Verification items for the finished model (mm, model axes). Face numbers are marked on the shaded views. A direction names the side the tool comes from. Round coordinates to 2 decimals unless told otherwise and drop trailing zeros. Loops run counter-clockwise (first coordinate to the right, second up) from the corner with the lowest first, then second, coordinate; pieces in that order, holes last. Notation, with made-up numbers: (27, 72.5) -> (80, 72.5) arc R17 ccw to (80, 88.5) -> close; hole circle Ø10 at (86.25, 54.5). An arc over 180 degrees is marked (long way). Use CSV: the item, a comma, the result in double quotes. Start each with the question number.
```python
from build123d import *

# Parameters (mm, degrees)
EXTRUDE_1_DEPTH     = 10
SKETCH_2_W          = 24
SKETCH_2_H          = 25
EXTRUDE_2_DEPTH     = 12
EXTRUDE_3_DEPTH     = 11
CUT_EXTRUDE_1_DEPTH = 15
SKETCH_5_W          = 15
SKETCH_5_H          = 17
CUT_EXTRUDE_2_DEPTH = 1
FILLET_2_R          = 12
FILLET_3_R          = 5
SKETCH_6_R          = 2.1
CUT_EXTRUDE_3_DEPTH = 30
CUT_EXTRUDE_START   = -15
SKETCH_7_R          = 3.5
CUT_EXTRUDE_4_DEPTH = 10


with BuildPart() as part:
    # 草图1 → 凸台-拉伸1 (new body)
    with BuildSketch(Plane.XY):
        Polygon((-7.5, 0), (-12, 0), (-12, -36), (12, -36), (12, 0), (7.5, 0), (7.5, -11), (-7.5, -11), align=None)
    extrude(amount=EXTRUDE_1_DEPTH)

    # 草图2 → 凸台-拉伸2 (add)
    with BuildSketch(Plane(origin=(0, 0, 0), x_dir=(-1, 0, 0), z_dir=(0, 0, -1))):
        with Locations((0, -23.5)):
            Rectangle(SKETCH_2_W, SKETCH_2_H)
    extrude(amount=EXTRUDE_2_DEPTH)

    # 草图3 → 凸台-拉伸3 (add)
    with BuildSketch(Plane(origin=(0, -11, 0), x_dir=(1, 0, 0), z_dir=(0, 1, 0))):
        Polygon((-7.5, 0), (-7.5, 7), (7.5, 7), (7.5, 0), (12, 0), (12, 12), (-12, 12), (-12, 0), align=None)
    extrude(amount=EXTRUDE_3_DEPTH)

    # 草图4 → 切除-拉伸1 (cut, symmetric)
    with BuildSketch(Plane(origin=(0, 0, 0), x_dir=(0, 0, -1), z_dir=(1, 0, 0))):
        Polygon((-1.382312477, 0), (12, -2), (12, 0), align=None)
    extrude(amount=CUT_EXTRUDE_1_DEPTH, both=True, mode=Mode.SUBTRACT)

    # 草图5 → 切除-拉伸2 (cut)
    with BuildSketch(Plane(origin=(0, -11, 0), x_dir=(1, 0, 0), z_dir=(0, 1, 0))):
        with Locations((0, -1.5)):
            Rectangle(SKETCH_5_W, SKETCH_5_H)
    extrude(amount=-CUT_EXTRUDE_2_DEPTH, mode=Mode.SUBTRACT)

    # 圆角2
    fillet_2_edges = [part.edges().sort_by_distance(p)[0] for p in [
        (12, -19, -12),
        (-12, -19, -12),
    ]]
    fillet(fillet_2_edges, radius=FILLET_2_R - 0.0001)  # a hair under: the kernel refuses the full size

    # 圆角3
    fillet_3_edges = [part.edges().sort_by_distance(p)[0] for p in [
        (8.485310664, -36, -8.485310664),
        (-8.485310664, -36, -8.485310664),
        (12, -36, 4.99995),
        (-12, -36, 4.99995),
    ]]
    fillet(fillet_3_edges, radius=FILLET_3_R)

    # 草图6 → 切除-拉伸3 (cut)
    with BuildSketch(Plane.XY.offset(10)):
        with Locations((4, -16)):
            Circle(SKETCH_6_R)
        with Locations((-4, -16)):
            Circle(SKETCH_6_R)
    extrude(amount=-CUT_EXTRUDE_3_DEPTH, mode=Mode.SUBTRACT)

    # 草图7 → 切除-拉伸4 (cut)
    with BuildSketch(Plane.XY.offset(10).offset(CUT_EXTRUDE_START)):
        with Locations((4, -16)):
            Circle(SKETCH_7_R)
        with Locations((-4, -16)):
            Circle(SKETCH_7_R)
    extrude(amount=-CUT_EXTRUDE_4_DEPTH, mode=Mode.SUBTRACT)


solid = part.part
```
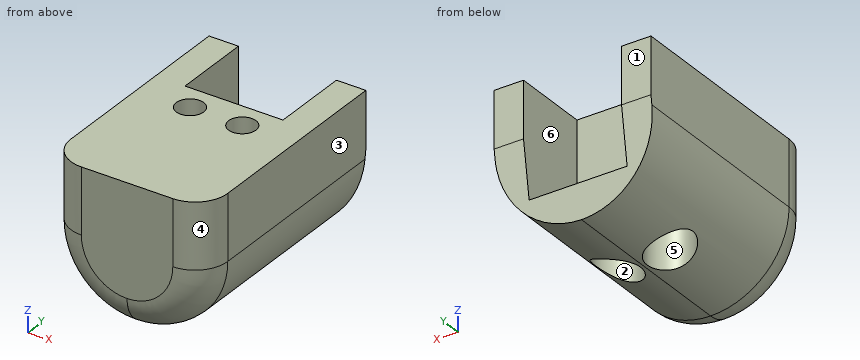
Q1. Depth check by flat-ended pin: pin 1 Ø2 at (x, y) = (-2.5, -15.5) entering from -Z; pin 2 Ø6 at (y, z) = (-23.5, -7) entering from -X; pin 3 Ø5.5 at (x, y) = (3.5, -4) entering from +Z. Enter the tip coordinate at first touch or a pass-through.
Q2. Thickness scan on L1, parallel to Y at x = 4, z = 5; L2, parallel to X at y = -16, z = -7.25; L3, parallel to Y at x = -6.5, z = -0.75. Record the ranges inside material, lowest first. Write a range as from..to.
Q3. Cross-section at A-A (z = 4.5). Record the boundary of the cut face in (x, y), and give its area (3 significant figures).
Q4. Tool access check on the marked faces 4, 5 and 6. Record the directions out of +Z, -Z, +X, -X, +Y, -Y that give a thin tool (end or side, any length) a straight path to the whole face; none if there is none.
Q5. Release check for a two-part mould opening along X. For the marked faces 1, 2 and 3 record: +X half, -X half, draft (parallel to the pull), parting line (faces both ways), or undercut.
Q6. Cross-section at C-C (y = -16). State how many separate pieces and enclosed holes the cut face has, and give its area (3 significant figures).
Answer list:
1,pin 1,"stops at z = -5"
1,pin 2,"stops at x = -11.31"
1,pin 3,"stops at z = -7"
2,L1,"y = -36..-18.1, -13.9..-12"
2,L2,"x = -9.56..-7.5, -0.5..0.5, 7.5..9.56"
2,L3,"y = -36..-12"
3,outline,"(-12, -31) arc R5 ccw to (-7, -36) -> (7, -36) arc R5 ccw to (12, -31) -> (12, 0) -> (7.5, 0) -> (7.5, -12) -> (-7.5, -12) -> (-7.5, 0) -> (-12, 0) -> close; hole circle Ø4.2 at (-4, -16); hole circle Ø4.2 at (4, -16)"
3,area,"646 mm2"
4,face 4,"+Z, -Z, +X, -Y"
4,face 5,"-Z"
4,face 6,"+Z, +Y"
5,face 1,"draft"
5,face 2,"undercut"
5,face 3,"+X half"
6,separate pieces,"3"
6,enclosed holes,"0"
6,area,"255 mm2"
